```python
from build123d import *

# Parameters (mm, degrees)
BOSS_EXTRUDE2_DEPTH  = 609.6
CUT_EXTRUDE1_DEPTH   = 1016
M6_CLEARANCE_HOLE1_D = 6.4


with BuildPart() as part:
    # Sketch3 → Boss-Extrude2 (new, symmetric)
    with BuildSketch(Plane.XY):
        Polygon((-15.875, 12.7), (-15.875, -12.7), (15.875, -12.7), (15.875, 12.7), (12.7, 12.7), (12.7, -9.525), (-12.7, -9.525), (-12.7, 12.7), align=None)
    extrude(amount=BOSS_EXTRUDE2_DEPTH, both=True)

    # Sketch5 → Cut-Extrude1 (cut)
    with BuildSketch(Plane.XY.offset(609.6)):
        Polygon((-15.875, 12.7), (-12.7, 12.7), (-12.7, -9.525), (12.7, -9.525), (12.7, 12.7), (15.875, 12.7), (15.875, -12.7), (-15.875, -12.7), align=None)
    extrude(amount=-CUT_EXTRUDE1_DEPTH, mode=Mode.SUBTRACT)

    # M6 Clearance Hole1 (through all)
    with Locations(Plane(origin=(0, -9.525, 0), x_dir=(1, 0, 0), z_dir=(0, 1, 0))):
        with Locations((0, 594.6)):
            Hole(M6_CLEARANCE_HOLE1_D / 2)


solid = part.part
```
Build history of the part. All positions in model axes, mm. A direction names the side the tool comes from. Coordinates: 2 decimals unless noted, no trailing zeros. Write each loop counter-clockwise with the first axis right and the second up, starting at its lowest first coordinate (ties: lowest second). Pieces come first, ordered by that corner, then holes.
1. Band-saw the part on B-B, the plane x = 0. Give the cut face in (y, z) (3 decimals).
Answer block:
outline: (-12.7, -609.6) - (-9.525, -609.6) - (-9.525, -597.8) - (-12.7, -597.8) - close; (-12.7, -591.4) - (-9.525, -591.4) - (-9.525, -406.4) - (-12.7, -406.4) - close
2. Band-saw the part on A-A, the plane z = -594.6. Give the cut face in (x, y) (3 decimals).
Answer block:
outline: (-15.875, -12.7) - (-3.2, -12.7) - (-3.2, -9.525) - (-12.7, -9.525) - (-12.7, 12.7) - (-15.875, 12.7) - close; (3.2, -12.7) - (15.875, -12.7) - (15.875, 12.7) - (12.7, 12.7) - (12.7, -9.525) - (3.2, -9.525) - close
3. Drop a flat-ended pin along its axis: pin 1 (7.5 mm diameter, centred on x = 2.5, z = -471, fed in from +Y) (3 decimals). Give the stop position or say it passes through.
Answer block:
pin 1: stops at y = -9.525
4. Band-saw the part on D-D, the plane z = -428. Give the cut face in (x, y) (3 decimals), and give its area (3 significant figures).
Answer block:
outline: (-15.875, -12.7) - (15.875, -12.7) - (15.875, 12.7) - (12.7, 12.7) - (12.7, -9.525) - (-12.7, -9.525) - (-12.7, 12.7) - (-15.875, 12.7) - close
area: 242 mm2
5. 3-axis set-ups, long thin cutter, end or side, ignore diameter. For faces 1 (the flat face through (15.875, 0, -507)), 2 (the flat face through (-12.7, 1, -507)): which of +Z, -Z, +X, -X, +Y, -Y reach the whole face in a straight line?
Answer block:
face 1: +Z, -Z, +X, +Y, -Y
face 2: +Z, -Z, +Y
6. Drill centre lines: probe 1 along X at (y, z) = (-11.7, -594.6) (3 decimals); probe 2 along X at (y, z) = (1.25, -516) (3 decimals); probe 3 along Z at (x, y) = (0, -11.5). Where is each one in solid material? Low to high.
Answer block:
probe 1: x = -15.875 to -3.2, 3.2 to 15.875
probe 2: x = -15.875 to -12.7, 12.7 to 15.875
probe 3: z = -609.6 to -597.8, -591.4 to -406.4
7. Pull direction Z, two halves, no side cores. Call faces 3 (the flat face through (0, -10, -406.4)), 4 (the flat face through (-15.875, 0, -507)), 5 (the flat face through (0, -10, -609.6)), 6 (the cylindrical face through (0.694, -11.135, -591.476)): released by +Z, released by -Z, zero draft, split by the parting line, or undercut.
Answer block:
face 3: released by +Z
face 4: zero draft
face 5: released by -Z
face 6: undercut
8. Band-saw the part on C-C, the plane y = 1.75. Give the cut face in (x, z) (3 decimals).
Answer block:
outline: (-15.875, -609.6) - (-12.7, -609.6) - (-12.7, -406.4) - (-15.875, -406.4) - close; (12.7, -609.6) - (15.875, -609.6) - (15.875, -406.4) - (12.7, -406.4) - close
